The figure shows three views and two pictorial views of one solid part (mm, origin at its lowest corner). Answer the questions. Coordinates: 2 decimals unless noted, no trailing zeros. Loops run counter-clockwise (first coordinate to the right, second up) from the corner with the lowest first, then second, coordinate; pieces in that order, holes last.
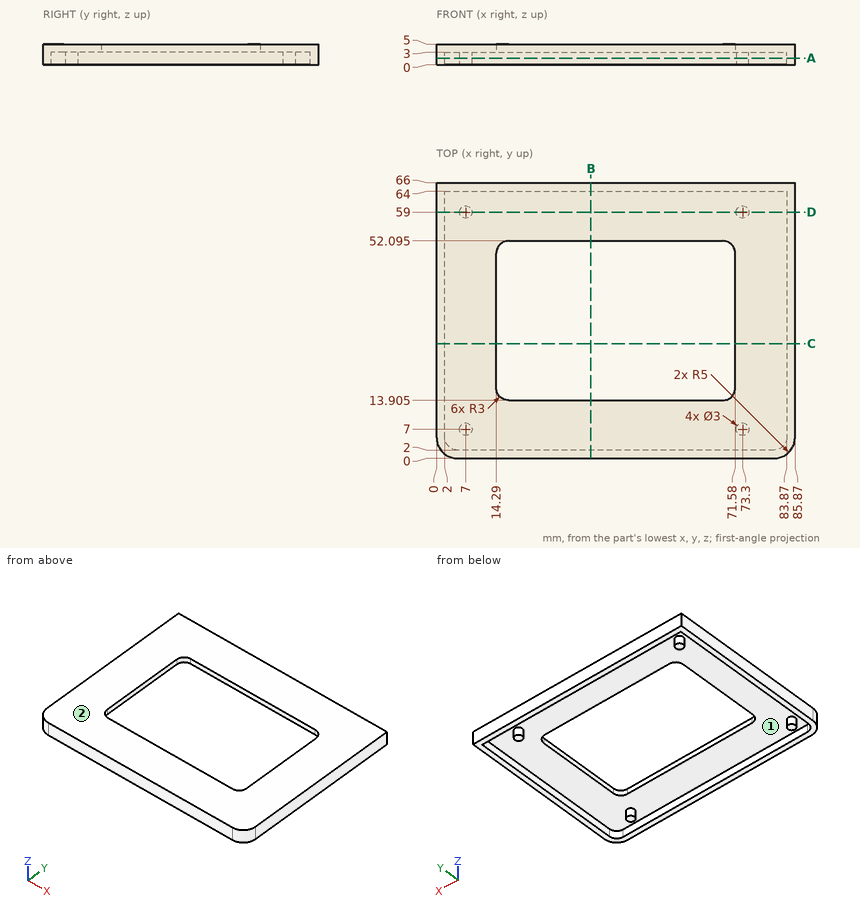
Q1. A flat-ended cylindrical pin translates along its axis: pin 1 Ø6 at (x, y) = (65.5, 55) entering from -Z. Find the tip coordinate at first contact, or state that the pin passes through.
Findings below:
pin 1: stops at z = 3
Q2. A cutting plane is placed at B-B (x = 37). Give the vertices of the cut face in (y, z) (3 decimals), then the cut area to 3 significant figures.
Findings below:
outline: (0, 0) - (2, 0) - (2, 3) - (13.905, 3) - (13.905, 5) - (0, 5) - close; (52.095, 3) - (64, 3) - (64, 0) - (66, 0) - (66, 5) - (52.095, 5) - close
area: 67.6 mm2
Q3. Straight lines are drawn through the part: probe 1 along Y at (x, z) = (56.5, 2.45); probe 2 along X at (y, z) = (37, 3.3); probe 3 along Y at (x, z) = (36, 4.75) (3 decimals). For each, find the intervals that lie inside material, in ascending order.
Findings below:
probe 1: y = 0 to 2, 64 to 66
probe 2: x = 0 to 14.29, 71.58 to 85.87
probe 3: y = 0 to 13.905, 52.095 to 66
Q4. A cutting plane is placed at C-C (y = 27.5). Give the vertices of the cut face in (x, z), then the cut area to 3 significant figures.
Findings below:
outline: (0, 0) - (2, 0) - (2, 3) - (14.29, 3) - (14.29, 5) - (0, 5) - close; (71.58, 3) - (83.87, 3) - (83.87, 0) - (85.87, 0) - (85.87, 5) - (71.58, 5) - close
area: 69.2 mm2
Q5. A cutting plane is placed at D-D (y = 59). Give the vertices of the cut face in (x, z).
Findings below:
outline: (0, 0) - (2, 0) - (2, 3) - (5.5, 3) - (5.5, 0) - (8.5, 0) - (8.5, 3) - (71.8, 3) - (71.8, 0) - (74.8, 0) - (74.8, 3) - (83.87, 3) - (83.87, 0) - (85.87, 0) - (85.87, 5) - (0, 5) - close
Q6. Determine the mould class of the marked faces 1 and 2 for opening direction X: +X half, -X half, draft (parallel to the pull), parting line (faces both ways), or undercut.
Findings below:
face 1: undercut
face 2: draft
Q7. A cutting plane is placed at A-A (z = 1.6). Give the vertices of the cut face in (x, y), then the cut area to 3 significant figures.
Findings below:
outline: (0, 5) arc R5 ccw to (5, 0) - (80.87, 0) arc R5 ccw to (85.87, 5) - (85.87, 66) - (0, 66) - close; circle Ø3 at (7, 7); circle Ø3 at (7, 59); circle Ø3 at (73.3, 7); circle Ø3 at (73.3, 59); hole (2, 5) arc R3 ccw to (5, 2) - (80.87, 2) arc R3 ccw to (83.87, 5) - (83.87, 64) - (2, 64) - close
area: 613 mm2
